from build123d import *

# Parameters (mm, degrees)
ESQUISSE1_W             = 45
ESQUISSE1_H             = 80
BOSS_EXTRU_1_DEPTH      = 1.5
CHANFREIN1_SIZE         = 8
ESQUISSE2_R             = 3
ENL_V_MAT_EXTRU_1_DEPTH = 2.5


with BuildPart() as part:
    # Esquisse1 → Boss.-Extru.1 (new body)
    with BuildSketch(Plane.XY):
        with Locations((22.5, 40)):
            Rectangle(ESQUISSE1_W, ESQUISSE1_H)
    extrude(amount=BOSS_EXTRU_1_DEPTH)

    # Chanfrein1
    chanfrein1_edges = [part.edges().sort_by_distance(p)[0] for p in [
        (0, 80, 0.75),
        (45, 80, 0.75),
        (45, 0, 0.75),
        (0, 0, 0.75),
    ]]
    chamfer(chanfrein1_edges, length=CHANFREIN1_SIZE)

    # Esquisse2 → Enlèv. mat.-Extru.1 (cut, through all)
    with BuildSketch(Plane.XY.offset(1.5)):
        with Locations((22.5, 75.9)):
            Circle(ESQUISSE2_R)
        with Locations((22.5, 4.1)):
            Circle(ESQUISSE2_R)
    extrude(amount=-ENL_V_MAT_EXTRU_1_DEPTH, mode=Mode.SUBTRACT)


solid = part.part
Model file for the job. Use its own axes, mm. Give positions to 0.01 mm unless a question says otherwise; leave off trailing zeros. Write each loop counter-clockwise with the first axis right and the second up, starting at its lowest first coordinate (ties: lowest second). Pieces come first, ordered by that corner, then holes. Notation, with made-up numbers: (87, -22) -> (128, -22) arc R24 ccw to (128, -8) -> close; hole circle Ø3 at (52, -2). An arc over 180 degrees is marked (long way). Write item = value, one per line.
(1) Mould opens along X. For faces 1 (the face through (22, 41, 0)), 2 (the face through (4, 76, 1)), 3 (the face through (45, 40, 1)), 4 (the face through (19.5, 4.2, 0.8)) say: released by +X, released by -X, zero draft, split by the parting line, or undercut.
Determined:
face_1 = zero draft
face_2 = released by -X
face_3 = released by +X
face_4 = undercut
(2) Probe line 1 along Y through (x, z) = (22.5, 0.65); line 2 along Y through (x, z) = (42.5, 1); line 3 along Y through (x, z) = (3, 0.7). List the from-to ranges inside material, lowest first.
Determined:
line_1 = 0 to 1.1, 7.1 to 72.9, 78.9 to 80
line_2 = 5.5 to 74.5
line_3 = 5 to 75
(3) Slice it at A-A, the plane z = 0.5. Give the cut face in (x, y).
Determined:
outline = (0, 8) -> (8, 0) -> (37, 0) -> (45, 8) -> (45, 72) -> (37, 80) -> (8, 80) -> (0, 72) -> close; hole circle Ø6 at (22.5, 4.1); hole circle Ø6 at (22.5, 75.9)
(4) Slice it at C-C, the plane y = 4.1. Give the cut face in (x, z), then the cut area to 3 significant figures.
Determined:
outline = (3.9, 0) -> (19.5, 0) -> (19.5, 1.5) -> (3.9, 1.5) -> close; (25.5, 0) -> (41.1, 0) -> (41.1, 1.5) -> (25.5, 1.5) -> close
area = 46.8 mm2
(5) Flat gauge pin, fed straight in: P1, Ø3.5, axis at x = 22.5, y = 75.9, coming from the +Z side. Where does the tip first touch, or does it go through?
Determined:
P1 = through
(6) Slice it at D-D, the plane x = 42. Give the cut face in (y, z).
Determined:
outline = (5, 0) -> (75, 0) -> (75, 1.5) -> (5, 1.5) -> close
(7) Slice it at B-B, the plane x = 22.5. Give the cut face in (y, z).
Determined:
outline = (0, 0) -> (1.1, 0) -> (1.1, 1.5) -> (0, 1.5) -> close; (7.1, 0) -> (72.9, 0) -> (72.9, 1.5) -> (7.1, 1.5) -> close; (78.9, 0) -> (80, 0) -> (80, 1.5) -> (78.9, 1.5) -> close
